Here's how the part is built. I have some questions about the finished solid (model axes, mm). Coordinates: 2 decimals unless noted, no trailing zeros. Loops run counter-clockwise (first coordinate to the right, second up) from the corner with the lowest first, then second, coordinate; pieces in that order, holes last. Notation, with made-up numbers: (60.25, 78) - (66.25, 78) arc R19 ccw to (66.25, 96) - close; hole circle Ø6 at (8.25, -39.5). An arc over 180 degrees is marked (long way). Use a Markdown table: item, result.
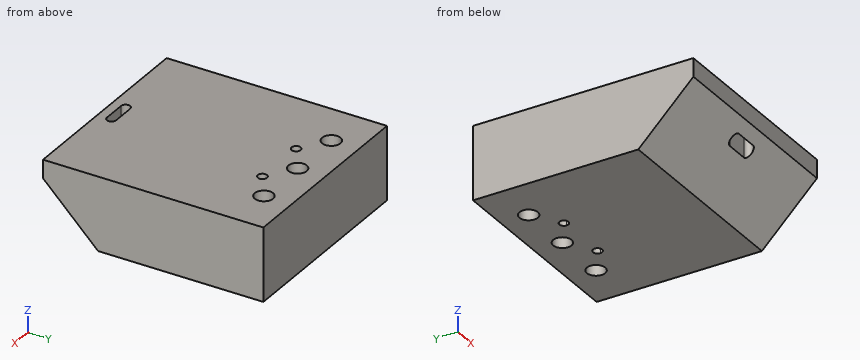
```python
from build123d import *

# Parameters (mm, degrees)
F0_W     = 139.7
F0_H     = 152.4
F1_DEPTH = 50.8
F2_R     = 6.35
F3_DEPTH = 50.801
F5_DEPTH = 139.701


with BuildPart() as f1:
    # F0 (on Top) → F1 (new body)
    with BuildSketch(Plane.XY):
        Rectangle(F0_W, F0_H)
    extrude(amount=-F1_DEPTH)

    # F2 (on face) → F3 (cut, through all)
    with BuildSketch(Plane.XY):
        with BuildLine():
            Line((-7.9375, -69.85), (7.9375, -69.85))
            ThreePointArc((7.9375, -69.85), (11.1125, -66.675), (7.9375, -63.5))
            Line((7.9375, -63.5), (-7.9375, -63.5))
            ThreePointArc((-7.9375, -63.5), (-11.1125, -66.675), (-7.9375, -69.85))
        make_face()
        with BuildLine():
            Line((0, 57.15), (6.35, 57.15))
            ThreePointArc((6.35, 57.15), (0, 63.5), (-6.35, 57.15))
            Line((-6.35, 57.15), (0, 57.15))
        make_face()
        with BuildLine():
            ThreePointArc((-15.875, 44.45), (-16.804936, 46.695064), (-19.05, 47.625))
            ThreePointArc((-19.05, 47.625), (-21.295064, 42.204936), (-15.875, 44.45))
        make_face()
        with Locations((-38.1, 57.15)):
            Circle(F2_R)
        with BuildLine():
            ThreePointArc((44.45, 57.15), (38.1, 63.5), (31.75, 57.15))
            ThreePointArc((31.75, 57.15), (38.1, 50.8), (44.45, 57.15))
        make_face()
        with BuildLine():
            ThreePointArc((22.225, 44.45), (21.295064, 46.695064), (19.05, 47.625))
            ThreePointArc((19.05, 47.625), (16.804936, 42.204936), (22.225, 44.45))
        make_face()
        with BuildLine():
            ThreePointArc((-6.35, 57.15), (0, 50.8), (6.35, 57.15))
            Line((6.35, 57.15), (0, 57.15))
            Line((0, 57.15), (-6.35, 57.15))
        make_face()
    extrude(amount=-F3_DEPTH, mode=Mode.SUBTRACT)

    # F4 (on face) → F5 (cut, through all)
    with BuildSketch(Plane.YZ.offset(69.85)):
        Polygon((-76.2, -12.7), (-76.2, -50.8), (-38.1, -50.8), align=None)
    extrude(amount=-F5_DEPTH, mode=Mode.SUBTRACT)


solid = f1.part
```
Q1. Will this pin go through, and if not, where does the flat tip stop? P1, Ø10, axis at x = 37, y = -47.5, coming from the -Z side.
Check values:
| item | result |
|---|---|
| P1 | z = -46.4 |
Q2. I want a section at C-C, the plane x = 0. Write out the boundary of the cut face in (y, z), then the cut area to 3 significant figures.
Check values:
| item | result |
|---|---|
| outline | (-76.2, -12.7) - (-69.85, -19.05) - (-69.85, 0) - (-76.2, 0) - close; (-63.5, -25.4) - (-38.1, -50.8) - (50.8, -50.8) - (50.8, 0) - (-63.5, 0) - close; (63.5, -50.8) - (76.2, -50.8) - (76.2, 0) - (63.5, 0) - close |
| area | 6,230 mm^2 |
Q3. Please list where these lines run through material, in increasing order: L1, parallel to Y at x = 0, z = -12; L2, parallel to X at y = 53.5, z = -23; L3, parallel to X at y = 45.5, z = -12.5. Write a range as from..to.
Check values:
| item | result |
|---|---|
| L1 | -76.2..-69.85, -63.5..50.8, 63.5..76.2 |
| L2 | -69.85..-43.3, -32.9..-5.2, 5.2..32.9, 43.3..69.85 |
| L3 | -69.85..-22.05, -16.05..16.05, 22.05..69.85 |
Q4. I want a section at B-B, the plane z = -5. Give the number of separate pieces and of enclosed holes in the cut face, then the cut area to 3 significant figures.
Check values:
| item | result |
|---|---|
| separate pieces | 1 |
| enclosed holes | 6 |
| area | 20,700 mm^2 |
Q5. I want a section at A-A, the plane x = 38.1. Write out the boundary of the cut face in (y, z), then the cut area to 3 significant figures.
Check values:
| item | result |
|---|---|
| outline | (-76.2, -12.7) - (-38.1, -50.8) - (50.8, -50.8) - (50.8, 0) - (-76.2, 0) - close; (63.5, -50.8) - (76.2, -50.8) - (76.2, 0) - (63.5, 0) - close |
| area | 6,370 mm^2 |
Q6. I want a section at D-D, the plane y = 57.15. Write out the boundary of the cut face in (x, z), then the cut area to 3 significant figures.
Check values:
| item | result |
|---|---|
| outline | (-69.85, -50.8) - (-44.45, -50.8) - (-44.45, 0) - (-69.85, 0) - close; (-31.75, -50.8) - (-6.35, -50.8) - (-6.35, 0) - (-31.75, 0) - close; (6.35, -50.8) - (31.75, -50.8) - (31.75, 0) - (6.35, 0) - close; (44.45, -50.8) - (69.85, -50.8) - (69.85, 0) - (44.45, 0) - close |
| area | 5,160 mm^2 |
